For this review, take the finished solid that the model builds, in its own axes (mm). Face numbers are marked on the shaded views. Coordinates: 2 decimals unless noted, no trailing zeros. Write each loop counter-clockwise with the first axis right and the second up, starting at its lowest first coordinate (ties: lowest second). Pieces come first, ordered by that corner, then holes.
1) We need section B-B on z = 217.25. Write out the cut boundary in (x, y), then the cut area to 3 significant figures.
2) We need section D-D on z = 213.5. Write out the cut boundary in (x, y), then the cut area to 3 significant figures.
3) Insertion check: P1, Ø1, axis at x = -0.5, y = 86.5, coming from the -Z side. The pin has a flat end and moves straight along its axis. Give the tip position at first contact, or say it passes through.
4) We need section C-C on x = -5. Write out the cut boundary in (y, z).
5) Mouldability with a two-part tool opening along Y and no side actions: class the marked faces 1, 2 and 3 as pulls with the +Y half, pulls with the -Y half, needs draft (parallel to the pull), parting line crosses it, or undercut.
6) To check wall thickness, follow line 1 along Y through (x, z) = (-5, 218.5); line 2 along Y through (x, z) = (-5, 220.5); line 3 along Y through (x, z) = (-1.75, 217.5). State the ranges of each line that lie inside material, in increasing order.
7) We need section A-A on y = 112. Write out the cut boundary in (x, z), then the cut area to 3 significant figures.
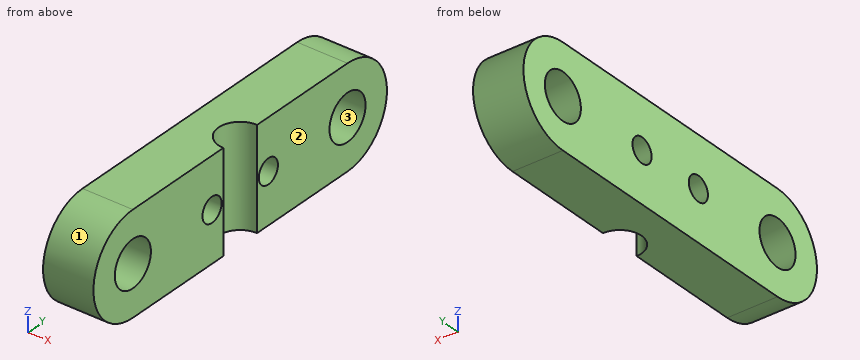
Solid Edge part; units mm, degrees
sketch "Sketch1" plane through (0, 0, 0) normal (1, 0, 0) x (0, 1, 0)
  circle A0 centre (126.0526, 218.3294) radius 3.2
  line L0 (87.9474, 225.3294) -> (126.0526, 225.3294)
  line L1 (126.0526, 211.3294) -> (87.9474, 211.3294)
  arc A1 (87.9474, 211.3294) -> (87.9474, 225.3294) centre (87.9474, 218.3294) cw
  arc A2 (126.0526, 225.3294) -> (126.0526, 211.3294) centre (126.0526, 218.3294) cw
  circle A3 centre (87.9474, 218.3294) radius 3.2
extrude "Protrusion1" add sketch "Sketch1" against normal blind 7
sketch "Sketch2" plane through (-4, 107, 225.3294) normal (0, 0, 1) x (1, 0, 0)
  circle A0 centre (4, 0) radius 3
extrude "Cutout1" cut sketch "Sketch2" against normal through all
sketch "Sketch3" plane through (-7, 107, 218.3294) normal (-1, 0, 0) x (0, -1, 0)
  circle A0 centre (-5, 0) radius 1.7
  circle A1 centre (5, 0) radius 1.7
extrude "Cutout2" cut sketch "Sketch3" against normal through all
properties material "ABS Plastic, high impact"
Result:
1. outline: (-7, 81.03) - (0, 81.03) - (0, 84.93) - (-7, 84.93) - close; (-7, 90.96) - (0, 90.96) - (0, 100.69) - (-7, 100.69) - close; (-7, 103.31) - (0, 103.31) - (0, 104) arc R3 cw to (0, 110) - (0, 110.69) - (-7, 110.69) - close; (-7, 113.31) - (0, 113.31) - (0, 123.04) - (-7, 123.04) - close; (-7, 129.07) - (0, 129.07) - (0, 132.97) - (-7, 132.97) - close
1. area: 228 mm2
2. outline: (-7, 82.88) - (0, 82.88) - (0, 104) arc R3 cw to (0, 110) - (0, 131.12) - (-7, 131.12) - close
2. area: 324 mm2
3. P1: stops at z = 211.39
4. outline: (87.95, 211.33) - (126.05, 211.33) arc R7 ccw to (126.05, 225.33) - (87.95, 225.33) arc R7 ccw to start; hole circle Ø6.4 at (87.95, 218.33); hole circle Ø3.4 at (102, 218.33); hole circle Ø3.4 at (112, 218.33); hole circle Ø6.4 at (126.05, 218.33)
5. face 1: pulls with the -Y half
5. face 2: needs draft
5. face 3: undercut
6. line 1: y = 80.95 to 84.75, 91.14 to 100.31, 103.69 to 110.31, 113.69 to 122.86, 129.25 to 133.05
6. line 2: y = 81.29 to 85.6, 90.3 to 123.7, 128.4 to 132.71
6. line 3: y = 81 to 84.86, 91.04 to 100.52, 103.48 to 104.56, 109.44 to 110.52, 113.48 to 122.96, 129.14 to 133
7. outline: (-7, 211.33) - (0, 211.33) - (0, 216.63) - (-7, 216.63) - close; (-7, 220.03) - (0, 220.03) - (0, 225.33) - (-7, 225.33) - close
7. area: 74.2 mm2
